Geometry check sheet. Reference: the model listing, model coordinates, mm. A direction names the side the tool comes from. Give positions to 0.01 mm unless a question says otherwise; leave off trailing zeros. Write each loop counter-clockwise with the first axis right and the second up, starting at its lowest first coordinate (ties: lowest second). Pieces come first, ordered by that corner, then holes. Notation, with made-up numbers: (-13.75, 40.5) -> (8.25, 40.5) arc R21 cw to (8.25, 61.5) -> close; hole circle Ø9 at (77, -13.75). An arc over 180 degrees is marked (long way). One line per item, written item: value.
from build123d import *

# Parameters (mm, degrees)
PAD_DEPTH       = 2
SKETCH017_W     = 10
SKETCH017_H     = 10
PAD006_DEPTH    = 2
SKETCH018_W     = 10
SKETCH018_H     = 10
PAD007_DEPTH    = 10
SKETCH020_R     = 1.6
POCKET008_DEPTH = 9
POCKET009_DEPTH = 4


with BuildPart() as part:
    # Sketch → Pad (new body)
    with BuildSketch(Plane.XY):
        with BuildLine():
            Line((5, 0), (90, 0))
            ThreePointArc((90, 0), (93.535534, 1.464466), (95, 5))
            Line((95, 5), (95, 35))
            ThreePointArc((95, 35), (93.535534, 38.535534), (90, 40))
            Line((90, 40), (5, 40))
            ThreePointArc((5, 40), (1.464466, 38.535534), (0, 35))
            Line((0, 35), (0, 5))
            ThreePointArc((0, 5), (1.464466, 1.464466), (5, 0))
        make_face()
    extrude(amount=PAD_DEPTH)

    # Sketch017 (on Face10 of Pad) → Pad006 (join)
    with BuildSketch(Plane.XY.offset(2)):
        with Locations((-5, 21.75)):
            Rectangle(SKETCH017_W, SKETCH017_H)
        with Locations((85, -5)):
            Rectangle(SKETCH017_W, SKETCH017_H)
        with Locations((85, 45)):
            Rectangle(SKETCH017_W, SKETCH017_H)
    extrude(amount=-PAD006_DEPTH)

    # Sketch018 (on Face18 of Pad006) → Pad007 (join)
    with BuildSketch(Plane.XY.offset(2)):
        with Locations((-5, 21.75)):
            Rectangle(SKETCH018_W, SKETCH018_H)
        with Locations((85, -5)):
            Rectangle(SKETCH018_W, SKETCH018_H)
        with Locations((85, 45)):
            Rectangle(SKETCH018_W, SKETCH018_H)
    extrude(amount=PAD007_DEPTH)

    # Sketch020 (on Face29 of Pad007) → Pocket008 (cut)
    with BuildSketch(Plane.XY.offset(12)):
        with Locations((85, -5)):
            Circle(SKETCH020_R)
        with Locations((85, 45)):
            Circle(SKETCH020_R)
        with Locations((-5, 21.75)):
            Circle(SKETCH020_R)
    extrude(amount=-POCKET008_DEPTH, mode=Mode.SUBTRACT)

    # Sketch021 (on Face29 of Pocket008) → Pocket009 (cut)
    with BuildSketch(Plane.XY.offset(12)):
        Polygon((-3.5, 19.151924), (-2, 21.75), (-3.5, 24.348076), (-6.5, 24.348076), (-8, 21.75), (-6.5, 19.151924), align=None)
        Polygon((87.598076, 43.5), (87.598076, 46.5), (85, 48), (82.401924, 46.5), (82.401924, 43.5), (85, 42), align=None)
        Polygon((87.598076, -6.5), (87.598076, -3.5), (85, -2), (82.401924, -3.5), (82.401924, -6.5), (85, -8), align=None)
    extrude(amount=-POCKET009_DEPTH, mode=Mode.SUBTRACT)


solid = part.part
1) Sectioned sample at D-D on y = 9. Record the cut outline in (x, z).
Verdict:
outline: (0, 0) -> (95, 0) -> (95, 2) -> (0, 2) -> close
2) Sectioned sample at B-B on y = -5. Record the cut outline in (x, z).
Verdict:
outline: (80, 0) -> (90, 0) -> (90, 12) -> (87.6, 12) -> (87.6, 8) -> (86.6, 8) -> (86.6, 3) -> (83.4, 3) -> (83.4, 8) -> (82.4, 8) -> (82.4, 12) -> (80, 12) -> close
3) Depth check by flat-ended pin: pin 1 Ø2 at (x, z) = (55.5, 0.5) entering from +Y; pin 2 Ø3.5 at (x, y) = (84.5, 44.5) entering from +Z; pin 3 Ø6 at (x, y) = (66.5, 12.5) entering from +Z; pin 4 Ø6 at (x, z) = (25.5, 6) entering from -Y. Enter the tip coordinate at first touch or a pass-through.
Verdict:
pin 1: y = 40
pin 2: z = 8
pin 3: z = 2
pin 4: through
4) Mould release check, pull along X, two halves, no side actions. Record for faces 4 (the flat face through (95, 20, 1)), 5 (the flat face through (83.72, -2.74, 10.03)), 6 (the flat face through (-3, 24, 12)): released by +X, released by -X, zero draft, split by the parting line, or undercut.
Verdict:
face 4: released by +X
face 5: undercut
face 6: zero draft
5) Sectioned sample at A-A on z = 6.75. Record the cut outline in (x, y).
Verdict:
outline: (-10, 16.75) -> (0, 16.75) -> (0, 26.75) -> (-10, 26.75) -> close; (80, -10) -> (90, -10) -> (90, 0) -> (80, 0) -> close; (80, 40) -> (90, 40) -> (90, 50) -> (80, 50) -> close; hole circle Ø3.2 at (-5, 21.75); hole circle Ø3.2 at (85, -5); hole circle Ø3.2 at (85, 45)
6) Scan lines: probe 1 along Y at (x, z) = (85, 4.25); probe 2 along X at (y, z) = (45, 10); probe 3 along Z at (x, y) = (22.5, 2.5). Record each from-to range of solid material in increasing order.
Verdict:
probe 1: -10 to -6.6, -3.4 to 0, 40 to 43.4, 46.6 to 50
probe 2: 80 to 82.4, 87.6 to 90
probe 3: 0 to 2
7) Sectioned sample at C-C on x = -5. Record the cut outline in (y, z).
Verdict:
outline: (16.75, 0) -> (26.75, 0) -> (26.75, 12) -> (24.35, 12) -> (24.35, 8) -> (23.35, 8) -> (23.35, 3) -> (20.15, 3) -> (20.15, 8) -> (19.15, 8) -> (19.15, 12) -> (16.75, 12) -> close
8) Tool access check on faces 1 (the flat face through (86.28, -7.26, 10.03)), 2 (the flat face through (53, 20, 0)), 3 (the flat face through (-5, 26.75, 6)). Record the directions out of +Z, -Z, +X, -X, +Y, -Y that give a thin tool (end or side, any length) a straight path to the whole face; none if there is none.
Verdict:
face 1: +Z
face 2: -Z, +X, -X, +Y, -Y
face 3: +Z, -Z, -X, +Y
